Check sheet for the modelled part. Datum: model origin and axes. Units: mm. A direction names the side the tool comes from. Round coordinates to 2 decimals unless told otherwise and drop trailing zeros. Loops run counter-clockwise (first coordinate to the right, second up) from the corner with the lowest first, then second, coordinate; pieces in that order, holes last. Notation, with made-up numbers: (14, 69.25) - (48, 69.25) arc R14 cw to (48, 90.25) - close; hole circle Ø1 at (-31.75, 4.5). An arc over 180 degrees is marked (long way). Put each result on its own line as item: value. Start each with the question number.
Item 1: Section check A-A, the plane x = 202. Record the cut outline in (y, z).
Item 2: Material ranges on line 1 along Y through (x, z) = (241, 2.5); line 2 along Y through (x, z) = (189.5, 7.5); line 3 along Y through (x, z) = (129.5, 4.25), recorded low to high.
Item 3: Tool access check on faces 1 (the flat face through (200, 63.294, 8)), 2 (the flat face through (67.311, 37, 5)), 3 (the flat face through (180.311, -26, 5)), 4 (the flat face through (178.311, 99, 5)). Record the directions out of +Z, -Z, +X, -X, +Y, -Y that give a thin tool (end or side, any length) a straight path to the whole face; none if there is none.
Item 4: Gauge pin test, flat ends, axial feed: pin 1 Ø3 at (y, z) = (37, 3.5) entering from -X; pin 2 Ø5 at (y, z) = (-27, 2.5) entering from -X; pin 3 Ø3 at (y, z) = (-25.5, 5.5) entering from +X. Record the tip position at first contact, or that the pin passes through.
Item 5: Section check B-B, the plane z = 7.5. Give the number of separate pieces and of enclosed holes in the cut face, and give its area (3 significant figures).
Item 6: Section check C-C, the plane y = 18.5. Record the cut outline in (x, z), and give its area (3 significant figures).
Item 7: Draft check along Y on faces 5 (the flat face through (98, 103.624, 5)), 6 (the flat face through (211, -30.376, 5)), 7 (the flat face through (57.311, 66, 5)), 8 (the flat face through (109.311, 1, 8)). Enter one of: pulls with the +Y half, pulls with the -Y half, needs draft (parallel to the pull), parting line crosses it, or undercut.
Autodesk Inventor part; units mm, degrees
ref_plane "YZ Plane" through (0, 0, 0) normal (1, 0, 0) x (0, 1, 0)
ref_plane "XZ Plane" through (0, 0, 0) normal (0, 1, 0) x (-1, 0, 0)
ref_plane "XY Plane" through (0, 0, 0) normal (0, 0, 1) x (1, 0, 0)
sketch "Эскиз1" plane through (0, 0, 0) normal (0, 0, 1) x (1, 0, 0)
  line L0 (174.3111, 41.624) -> (229.3111, 41.624)
  line L1 (229.3111, 41.624) -> (229.3111, 31.624)
  line L2 (229.3111, 31.624) -> (174.3111, 31.624)
  line L3 (174.3111, 41.624) -> (174.3111, 31.624)
  line L4 (149.3111, 46.624) -> (159.3111, 46.624)
  line L5 (149.3111, 46.624) -> (149.3111, 86.624)
  line L6 (149.3111, 86.624) -> (159.3111, 86.624)
  line L7 (159.3111, 86.624) -> (159.3111, 46.624)
  line L8 (134.3111, 31.624) -> (134.3111, 41.624)
  line L9 (134.3111, 31.624) -> (79.3111, 31.624)
  line L10 (79.3111, 31.624) -> (79.3111, 41.624)
  line L11 (79.3111, 41.624) -> (134.3111, 41.624)
  line L12 (251.3111, -20.5639) -> (251.3111, 93.8118)
  arc A0 (241.499, 103.624) -> (251.3111, 93.8118) centre (247.0611, 99.374) ccw
  line L13 (241.499, 103.624) -> (180.3111, 103.624)
  line L14 (180.3111, 103.624) -> (180.3111, 94.124)
  line L15 (180.3111, 94.124) -> (178.3111, 94.124)
  line L16 (178.3111, 94.124) -> (178.3111, 103.624)
  line L17 (178.3111, 103.624) -> (130.3111, 103.624)
  line L18 (130.3111, 103.624) -> (130.3111, 94.124)
  line L19 (130.3111, 94.124) -> (128.3111, 94.124)
  line L20 (128.3111, 94.124) -> (128.3111, 103.624)
  line L21 (128.3111, 103.624) -> (67.1233, 103.624)
  arc A1 (57.3111, 93.8118) -> (67.1233, 103.624) centre (61.5611, 99.374) ccw
  line L22 (57.3111, -20.5639) -> (57.3111, 93.8118)
  arc A2 (67.1233, -30.376) -> (57.3111, -20.5639) centre (61.5611, -26.126) ccw
  line L23 (128.3111, -30.376) -> (67.1233, -30.376)
  line L24 (128.3111, -30.376) -> (128.3111, -20.876)
  line L25 (128.3111, -20.876) -> (130.3111, -20.876)
  line L26 (130.3111, -20.876) -> (130.3111, -30.376)
  line L27 (178.3111, -30.376) -> (130.3111, -30.376)
  line L28 (178.3111, -30.376) -> (178.3111, -20.876)
  line L29 (178.3111, -20.876) -> (180.3111, -20.876)
  line L30 (180.3111, -20.876) -> (180.3111, -30.376)
  line L31 (241.499, -30.376) -> (180.3111, -30.376)
  arc A3 (251.3111, -20.5639) -> (241.499, -30.376) centre (247.0611, -26.126) ccw
  circle A4 centre (229.3111, 86.624) radius 5
  circle A5 centre (79.3111, -13.376) radius 5
  circle A6 centre (79.3111, 86.624) radius 5
  circle A7 centre (229.3111, -13.376) radius 5
  line L32 (159.3111, 26.624) -> (149.3111, 26.624)
  line L33 (159.3111, 26.624) -> (159.3111, -13.376)
  line L34 (159.3111, -13.376) -> (149.3111, -13.376)
  line L35 (149.3111, -13.376) -> (149.3111, 26.624)
  line L36 (241.499, 103.624) -> (67.1233, 103.624)
  line L37 (57.3111, 93.8118) -> (57.3111, -20.5639)
  line L38 (67.1233, -30.376) -> (241.499, -30.376)
  line L39 (251.3111, -20.5639) -> (251.3111, 93.8118)
  arc A8 (251.3111, -20.5639) -> (241.499, -30.376) centre (247.0611, -26.126) ccw
  arc A9 (67.1233, -30.376) -> (57.3111, -20.5639) centre (61.5611, -26.126) ccw
  arc A10 (57.3111, 93.8118) -> (67.1233, 103.624) centre (61.5611, 99.374) ccw
  arc A11 (241.499, 103.624) -> (251.3111, 93.8118) centre (247.0611, 99.374) ccw
  line L40 (57.3111, 35.624) -> (57.3111, 37.624) construction
  line L41 (251.3111, 35.624) -> (251.3111, 37.624) construction
  line L42 (181.3111, -30.376) -> (177.3111, -30.376)
  line L43 (177.3111, -30.376) -> (177.3111, -20.376)
  line L44 (177.3111, -20.376) -> (181.3111, -20.376)
  line L45 (181.3111, -20.376) -> (181.3111, -30.376)
  line L46 (131.3111, -30.376) -> (127.3111, -30.376)
  line L47 (127.3111, -30.376) -> (127.3111, -20.376)
  line L48 (127.3111, -20.376) -> (131.3111, -20.376)
  line L49 (131.3111, -20.376) -> (131.3111, -30.376)
  line L50 (57.3111, 34.624) -> (67.3111, 34.624)
  line L51 (67.3111, 34.624) -> (67.3111, 38.624)
  line L52 (67.3111, 38.624) -> (57.3111, 38.624)
  line L53 (57.3111, 38.624) -> (57.3111, 34.624)
  line L54 (131.3111, 103.624) -> (127.3111, 103.624)
  line L55 (127.3111, 103.624) -> (127.3111, 93.624)
  line L56 (127.3111, 93.624) -> (131.3111, 93.624)
  line L57 (131.3111, 93.624) -> (131.3111, 103.624)
  line L58 (181.3111, 103.624) -> (177.3111, 103.624)
  line L59 (177.3111, 103.624) -> (177.3111, 93.624)
  line L60 (177.3111, 93.624) -> (181.3111, 93.624)
  line L61 (181.3111, 93.624) -> (181.3111, 103.624)
  line L62 (251.3111, 38.624) -> (241.3111, 38.624)
  line L63 (241.3111, 38.624) -> (241.3111, 34.624)
  line L64 (241.3111, 34.624) -> (251.3111, 34.624)
  line L65 (251.3111, 34.624) -> (251.3111, 38.624)
  point P0 (0, 0)
  point P1 (154.3111, 103.624)
  point P2 (154.3111, -30.376)
  point P3 (57.3111, 36.624)
  point P4 (251.3111, 36.624)
  point P5 (179.3111, -20.376)
  point P6 (179.3111, -20.876)
  point P7 (129.3111, -20.376)
  point P8 (129.3111, -20.876)
  point P9 (67.3111, 36.624)
  point P10 (66.8111, 36.624)
  point P11 (129.3111, 93.624)
  point P12 (129.3111, 94.124)
  point P13 (179.3111, 93.624)
  point P14 (179.3111, 94.124)
  point P15 (241.3111, 36.624)
  point P16 (241.8111, 36.624)
  dimension "d0" = 4
  dimension "d1" = 10
  dimension "d2" = 10
  dimension "d3" = 4
  dimension "d4" = 10
  dimension "d5" = 4
  dimension "d6" = 10
  dimension "d7" = 4
  dimension "d8" = 4
  dimension "d9" = 10
  dimension "d10" = 10
  dimension "d11" = 4
extrude "Выдавливание1" add sketch "Эскиз1" along normal blind 10 contours L0 L1 L2 L3 | L5 L6 L7 L4 | L9 L10 L11 L8 | A3 L31 L45 L44 L43 L27 L49 L48 L47 L23 A2 L22 L50 L51 L52 A1 L21 L55 L56 L57 L17 L59 L60 L61 L13 A0 L12 L62 L63 L64 | L64 L63 L62 L12 | L31 L30 L29 L28 L27 L43 L44 L45 | L61 L60 L59 L17 L16 L15 L14 L13 | A4 | A5 | A6 | A7 | L33 L34 L35 L32
sketch "Эскиз2" plane through (0, 0, 10) normal (0, 0, 1) x (1, 0, 0)
  line L0 (251.3111, 9.954) -> (149.7111, 9.954)
  line L1 (149.7111, 9.954) -> (149.7111, 63.294)
  line L2 (149.7111, 63.294) -> (251.3111, 63.294)
  line L3 (251.3111, 63.294) -> (251.3111, 9.954)
  line L4 (251.3111, -20.5639) -> (251.3111, 35.624)
  line L5 (251.3111, 37.624) -> (251.3111, 93.8118)
  line L6 (251.3111, 35.624) -> (251.3111, 37.624) construction
  line L7 (154.7911, 9.954) -> (251.3111, 9.954)
  point P0 (0, 0)
  point P1 (251.3111, 36.624)
  dimension "d14" = 101.6
  dimension "d15" = 53.34
extrude "Выдавливание2" cut sketch "Эскиз2" against normal blind 4
sketch "Эскиз9" plane through (0, 0, 10) normal (0, 0, 1) x (1, 0, 0)
  line L0 (109.3111, 83.624) -> (107.3111, 83.624)
  line L1 (109.3111, 62.124) -> (109.3111, 81.124)
  line L2 (107.3111, 62.124) -> (107.3111, 81.124)
  line L3 (109.3111, 59.624) -> (107.3111, 59.624)
  line L4 (106.4111, 62.5941) -> (106.4111, 64.4694)
  line L5 (106.4111, 69.3382) -> (106.4111, 70.0888)
  line L6 (106.4111, 77.7718) -> (106.4111, 78.6108)
  line L7 (106.4111, 79.5822) -> (106.4111, 80.2887)
  line L8 (109.3111, 83.624) -> (106.4111, 83.624)
  line L9 (106.4111, 83.624) -> (106.4111, 59.624)
  line L10 (106.4111, 59.624) -> (109.3111, 59.624)
  line L11 (109.3111, 59.624) -> (109.3111, 83.624)
  point P0 (0, 0)
extrude "Выдавливание11" cut sketch "Эскиз9" against normal blind 4
pattern_linear "Прямоуг.массив1" count 2 spacing 70 along (0, -1, 0) of "Выдавливание11"
equation "\"d2\" = d1"
equation "\"d3\" = d0"
equation "\"d4\" = d2"
equation "\"d5\" = d3"
equation "\"d6\" = d4"
equation "\"d7\" = d5"
equation "\"d8\" = d7"
equation "\"d9\" = d6"
equation "\"d10\" = d1"
equation "\"d11\" = d0"
properties part number "Каркас"
Check result:
1. outline: (-30.38, 0) - (103.62, 0) - (103.62, 10) - (63.29, 10) - (63.29, 6) - (9.95, 6) - (9.95, 10) - (-30.38, 10) - close
2. line 1: -30.38 to -29.63, -22.62 to 95.87, 102.88 to 103.62
2. line 2: -30.38 to 9.95, 63.29 to 103.62
2. line 3: -20.38 to 93.62
3. face 1: +Z, +X
3. face 2: +Z, -Z, -X
3. face 3: +Z, -Z, -Y
3. face 4: +Z, -Z, +Y
4. pin 1: x = 67.31
4. pin 2: x = 67.69
4. pin 3: x = 240.39
5. separate pieces: 1
5. enclosed holes: 2
5. area: 19,800 mm²
6. outline: (57.31, 0) - (251.31, 0) - (251.31, 6) - (149.71, 6) - (149.71, 10) - (57.31, 10) - close
6. area: 1,530 mm²
7. face 5: pulls with the +Y half
7. face 6: pulls with the -Y half
7. face 7: needs draft
7. face 8: undercut
